Input: part model. Units: mm. Frame: model coordinates. Face numbers are marked on the shaded views. A direction names the side the tool comes from. Coordinates: 2 decimals unless noted, no trailing zeros. Write each loop counter-clockwise with the first axis right and the second up, starting at its lowest first coordinate (ties: lowest second). Pieces come first, ordered by that corner, then holes. Notation, with made-up numbers: (-24, 37) - (4, 37) arc R7 cw to (4, 48) - close; hole circle Ø4 at (68.25, -21.5). An arc over 180 degrees is marked (long way). Use a Markdown table: item, result. Add a question column.
Q1. Section query C-C (y = -8.5). Give the number of separate pieces and of enclosed holes in the cut face, then the cut area to 3 significant figures.
Q2. Mould query, pull axis X, two halves, no side actions, for the marked faces 4, 5 and 6. Classes: released by +X, released by -X, zero draft, split by the parting line, or undercut.
Q3. Section query A-A (x = 5). Return the cut outline in (y, z) (3 decimals), then the cut area to 3 significant figures.
Q4. Set-up query: the marked faces 1, 2 and 3. Return all of +Z, -Z, +X, -X, +Y, -Y with unobstructed straight access to the full face (end or side cutting, diameter ignored); none if empty.
Q5. Material intervals for probe 1 along Z at (x, y) = (5, -1.25) (3 decimals); probe 2 along Z at (x, y) = (-19, 6.75); probe 3 along X at (y, z) = (-7, 0), sorted ascending. Write a range as from..to.
Q6. Pin query (flat end, axial travel): P1, Ø1, axis at y = 0.5, z = 0, coming from the +X side; P2, Ø2.5, axis at x = 17, z = -31.55, coming from the +Y side; P3, Ø3, axis at x = -19, z = -15, coming from the -Y side; P4, Ø2, axis at y = 1.5, z = -27.5, coming from the -X side. Return the tip coordinate at first contact, or that it passes through.
Q7. Section query B-B (z = -7.5). Return the cut outline in (x, y), then the cut area to 3 significant figures.
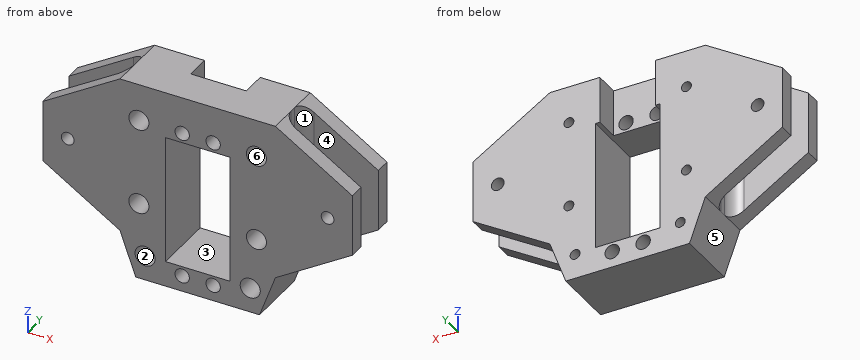
from build123d import *

# Parameters (mm, degrees)
MAIN_BODY_DEPTH           = 10
SKETCH2_R                 = 2.325
SKETCH2_R_2               = 2.0625
SKETCH2_W                 = 20.8
SKETCH2_H                 = 41.7
SERVO_ROTROD_CUTOUT_DEPTH = 30
SKETCH3_W                 = 18
SKETCH3_H                 = 8
SERVO_CABLE_CUTOUT_DEPTH  = 56.752305
CONTROL_ARM_CUTOUT_START  = -66
SKETCH4_W                 = 24.86969785
SKETCH4_H                 = 10
CONTROL_ARM_CUTOUT_DEPTH  = 67
FILLET1_R                 = 4
SKETCH6_R                 = 1.6
MOUNT_HOLES_CHASSIS_DEPTH = 21
SKETCH7_R                 = 3.25
BOLT_HEAD_HOLES_DEPTH     = 8


with BuildPart() as part:
    # Sketch1 → Main-Body (new body, symmetric)
    with BuildSketch(Plane(origin=(0, 0, 0), x_dir=(1, 0, 0), z_dir=(0, 1, 0))):
        Polygon((20, 39.547694656), (-20, 39.547694656), (-25.13030215, 25.452305344), (-50, 10), (-50, -10), (-25.13030215, -25.452305344), (25.13030215, -25.452305344), (50, -10), (50, 10), (25.13030215, 25.452305344), align=None)
    extrude(amount=MAIN_BODY_DEPTH, both=True)

    # Sketch2 → Servo&RotRod-Cutout (cut)
    with BuildSketch(Plane(origin=(0, 10, 0), x_dir=(1, 0, 0), z_dir=(0, 1, 0))):
        with Locations((-5, -13.5)):
            Circle(SKETCH2_R)
        with Locations((5, -13.5)):
            Circle(SKETCH2_R)
        with Locations((-5, 34.4)):
            Circle(SKETCH2_R)
        with Locations((5, 34.4)):
            Circle(SKETCH2_R)
        with Locations((-42, 0)):
            Circle(SKETCH2_R_2)
        with Locations((42, 0)):
            Circle(SKETCH2_R_2)
        with Locations((0, 10.45)):
            Rectangle(SKETCH2_W, SKETCH2_H)
    extrude(amount=-SERVO_ROTROD_CUTOUT_DEPTH, mode=Mode.SUBTRACT)

    # Sketch3 → Servo-Cable-Cutout (cut)
    with BuildSketch(Plane.XY.offset(25.452305344)):
        with Locations((0, 6)):
            Rectangle(SKETCH3_W, SKETCH3_H)
    extrude(amount=-SERVO_CABLE_CUTOUT_DEPTH, mode=Mode.SUBTRACT)

    # Sketch4 → Control-Arm-Cutout (cut)
    with BuildSketch(Plane.XY.offset(25.452305344).offset(CONTROL_ARM_CUTOUT_START)):
        with Locations((-37.565151075, 0)):
            Rectangle(SKETCH4_W, SKETCH4_H)
    control_arm_cutout = extrude(amount=CONTROL_ARM_CUTOUT_DEPTH, mode=Mode.SUBTRACT)

    # Mirror1: Control-Arm-Cutout across plane
    add(control_arm_cutout.mirror(Plane(origin=(0, 0, 0), x_dir=(0, 0, 1), z_dir=(1, 0, 0))), mode=Mode.SUBTRACT)

    # Fillet1
    fillet1_edges = [part.edges().sort_by_distance(p)[0] for p in [
        (-25.13030215, 5, 0),
        (-25.13030215, -5, 0),
        (25.13030215, -5, 0),
        (25.13030215, 5, 0),
    ]]
    fillet(fillet1_edges, radius=FILLET1_R)

    # Sketch6 → Mount-Holes-Chassis (cut, through all)
    with BuildSketch(Plane.XZ.offset(10)):
        with Locations((19, -14.547694656)):
            Circle(SKETCH6_R)
        with Locations((19, 13.452305344)):
            Circle(SKETCH6_R)
        with Locations((17, -31.547694656)):
            Circle(SKETCH6_R)
        with Locations((-17, -31.547694656)):
            Circle(SKETCH6_R)
        with Locations((-19, 13.452305344)):
            Circle(SKETCH6_R)
        with Locations((-19, -14.547694656)):
            Circle(SKETCH6_R)
    extrude(amount=-MOUNT_HOLES_CHASSIS_DEPTH, mode=Mode.SUBTRACT)

    # Sketch7 → Bolt-Head-Holes (cut)
    with BuildSketch(Plane.XZ.offset(10)):
        with Locations((17, -31.547694656)):
            Circle(SKETCH7_R)
        with Locations((19, -14.547694656)):
            Circle(SKETCH7_R)
        with Locations((19, 13.452305344)):
            Circle(SKETCH7_R)
        with Locations((-19, 13.452305344)):
            Circle(SKETCH7_R)
        with Locations((-19, -14.547694656)):
            Circle(SKETCH7_R)
        with Locations((-17, -31.547694656)):
            Circle(SKETCH7_R)
    extrude(amount=-BOLT_HEAD_HOLES_DEPTH, mode=Mode.SUBTRACT)


solid = part.part
Values follow:
| question | item | result |
|---|---|---|
| 1 | separate pieces | 1 |
| 1 | enclosed holes | 13 |
| 1 | area | 3,800 mm2 |
| 2 | face 4 | zero draft |
| 2 | face 5 | released by -X |
| 2 | face 6 | undercut |
| 3 | outline | (-10, -39.548) - (10, -39.548) - (10, -36.725) - (-10, -36.725) - close; (-10, -32.075) - (10, -32.075) - (10, -31.3) - (-10, -31.3) - close; (-10, 10.4) - (2, 10.4) - (2, 11.175) - (-10, 11.175) - close; (-10, 15.825) - (2, 15.825) - (2, 25.452) - (-10, 25.452) - close |
| 3 | area | 197 mm2 |
| 4 | face 1 | +Z, -Z, +X |
| 4 | face 2 | -Y |
| 4 | face 3 | +Y, -Y |
| 5 | probe 1 | -39.548..-36.725, -32.075..-31.3, 10.4..11.175, 15.825..25.452 |
| 5 | probe 2 | -39.55..-16.15, -12.95..11.85, 15.05..25.45 |
| 5 | probe 3 | -50..-44.06, -39.94..-10.4, 10.4..39.94, 44.06..50 |
| 6 | P1 | x = 25.13 |
| 6 | P2 | through |
| 6 | P3 | y = -2 |
| 6 | P4 | x = -24.75 |
| 7 | outline | (-50, -10) - (-10.4, -10) - (-10.4, 10) - (-50, 10) - (-50, 5) - (-29.13, 5) arc R4 cw to (-25.13, 1) - (-25.13, -1) arc R4 cw to (-29.13, -5) - (-50, -5) - close; (10.4, -10) - (50, -10) - (50, -5) - (29.13, -5) arc R4 cw to (25.13, -1) - (25.13, 1) arc R4 cw to (29.13, 5) - (50, 5) - (50, 10) - (10.4, 10) - close |
| 7 | area | 1,100 mm2 |
